Source: CAD feature listing. Evaluate the final solid. Frame: model axes, mm. Round coordinates to 2 decimals unless told otherwise and drop trailing zeros. Order: outer loops, then holes, each group sorted by start corner. A loop starts at its lowest first (then second) coordinate and runs counter-clockwise, first axis right, second up. Notation, with made-up numbers: (6, -21.5) -> (61, -21.5) arc R31 ccw to (61, 14.5) -> close; hole circle Ø8 at (6.5, 82.5). An arc over 180 degrees is marked (long way). Write item = value, one per line. Start each with the question number.
(1) Cut plane D-D on x = 5.5. Return the cut outline in (y, z), then the cut area to 3 significant figures.
(2) Cut plane B-B on z = -8.5. Return the cut outline in (x, y).
(3) Cut plane C-C on z = -1.25. Return the cut outline in (x, y).
(4) Ray query, line 1 (X direction, y = 2.15, z = -9.25); line 2 (Z direction, x = -12, y = 1.55); line 3 (X direction, y = 2.6, z = 9.25). Return the intervals inside material, ascending.
(5) Cut plane A-A on y = 1.85. Return the cut outline in (x, z), then the cut area to 3 significant figures.
from build123d import *

# Parameters (mm, degrees)
SKETCH1_W           = 43
SKETCH1_H           = 22
BOSS_EXTRUDE1_DEPTH = 2.8
SKETCH2_R           = 14
CUT_EXTRUDE1_DEPTH  = 25.312342544
FILLET1_R           = 2


with BuildPart() as part:
    # Sketch1 → Boss-Extrude1 (new body)
    with BuildSketch(Plane(origin=(0, 0, 0), x_dir=(1, 0, 0), z_dir=(0, 1, 0))):
        Rectangle(SKETCH1_W, SKETCH1_H)
    extrude(amount=BOSS_EXTRUDE1_DEPTH)

    # Sketch2 → Cut-Extrude1 (cut, through all)
    with BuildSketch(Plane(origin=(0, 2.8, 0), x_dir=(1, 0, 0), z_dir=(0, 1, 0))):
        with Locations((0, 14)):
            Circle(SKETCH2_R)
    extrude(amount=-CUT_EXTRUDE1_DEPTH, mode=Mode.SUBTRACT)

    # Fillet1
    fillet1_edges = [part.edges().sort_by_distance(p)[0] for p in [
        (21.5, 1.4, 11),
        (-21.5, 1.4, 11),
        (-21.5, 1.4, -11),
        (21.5, 1.4, -11),
    ]]
    fillet(fillet1_edges, radius=FILLET1_R)


solid = part.part
Evaluation:
q1.outline = (0, -1.13) -> (2.8, -1.13) -> (2.8, 11) -> (0, 11) -> close
q1.area = 34.0 mm^2
q2.outline = (-21.5, 0) -> (-12.87, 0) -> (-12.87, 2.8) -> (-21.5, 2.8) -> close; (12.87, 0) -> (21.5, 0) -> (21.5, 2.8) -> (12.87, 2.8) -> close
q3.outline = (-21.5, 0) -> (-5.78, 0) -> (-5.78, 2.8) -> (-21.5, 2.8) -> close; (5.78, 0) -> (21.5, 0) -> (21.5, 2.8) -> (5.78, 2.8) -> close
q4.line_1 = -21.48 to -13.17, 13.17 to 21.48
q4.line_2 = -6.79 to 11
q4.line_3 = -21.48 to 21.48
q5.outline = (-21.5, -9) arc R2 ccw to (-19.5, -11) -> (-13.67, -11) arc R14 cw to (13.67, -11) -> (19.5, -11) arc R2 ccw to (21.5, -9) -> (21.5, 9) arc R2 ccw to (19.5, 11) -> (-19.5, 11) arc R2 ccw to (-21.5, 9) -> close
q5.area = 718 mm^2
